Part print with two shaded views. Sizes in mm from the minimum x, y, z corner. Round coordinates to 2 decimals unless told otherwise and drop trailing zeros. Loops run counter-clockwise (first coordinate to the right, second up) from the corner with the lowest first, then second, coordinate; pieces in that order, holes last.
(1) Flat gauge pins, fed straight in: pin 1 (6.5 mm diameter, centred on y = 3.5, z = 109.5, fed in from -X); pin 2 (14 mm diameter, centred on y = 4, z = 96.5, fed in from +X); pin 3 (10 mm diameter, centred on x = 15.5, y = 299.5, fed in from -Z). Where does each tip first touch, or does it go through?
(2) Cut at A-A on y = 169.5. List the corners of the cut face in (x, z).
(3) Cut at B-B on z = 215. List the corners of the cut face in (x, y).
(4) Probe probe 1 along Z at (x, y) = (11, 170.5); probe 2 along Y at (x, z) = (1, 171.5); probe 3 along X at (y, z) = (194.5, 311.5). List the from-to ranges inside material, lowest first.
(5) Cut at C-C on z = 33. List the corners of the cut face in (x, y), then the cut area to 3 significant figures.
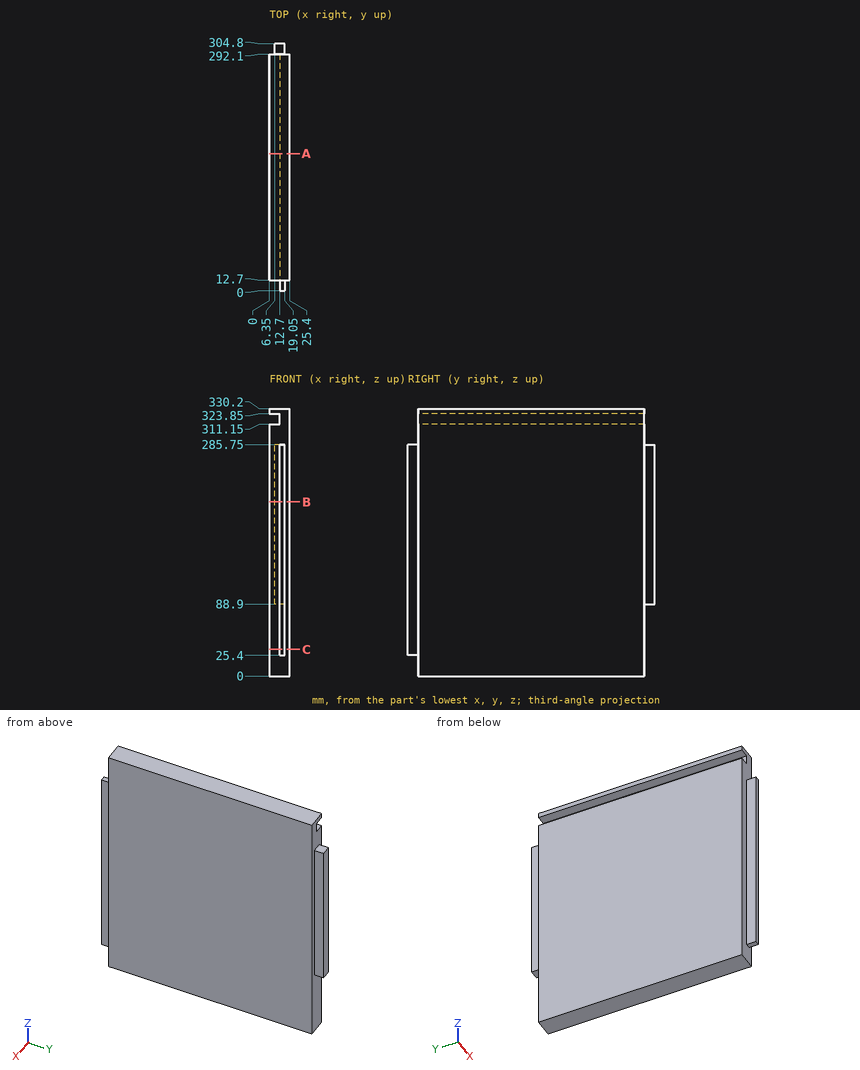
Final values:
1. pin 1: stops at x = 12.7
1. pin 2: stops at x = 19.05
1. pin 3: stops at z = 88.9
2. outline: (0, 0) - (25.4, 0) - (25.4, 330.2) - (0, 330.2) - (0, 323.85) - (12.7, 323.85) - (12.7, 311.15) - (0, 311.15) - close
3. outline: (0, 12.7) - (12.7, 12.7) - (12.7, 0) - (19.05, 0) - (19.05, 12.7) - (25.4, 12.7) - (25.4, 292.1) - (19.05, 292.1) - (19.05, 304.8) - (6.35, 304.8) - (6.35, 292.1) - (0, 292.1) - close
4. probe 1: z = 0 to 311.15, 323.85 to 330.2
4. probe 2: y = 12.7 to 292.1
4. probe 3: x = 12.7 to 25.4
5. outline: (0, 12.7) - (12.7, 12.7) - (12.7, 0) - (19.05, 0) - (19.05, 12.7) - (25.4, 12.7) - (25.4, 292.1) - (0, 292.1) - close
5. area: 7,180 mm2
